The model under review builds one solid part; all positions refer to its coordinate system, in mm. Round coordinates to 2 decimals unless told otherwise and drop trailing zeros. Loops run counter-clockwise (first coordinate to the right, second up) from the corner with the lowest first, then second, coordinate; pieces in that order, holes last. Notation, with made-up numbers: (42.5, 50) -> (83.5, 50) arc R22 ccw to (83.5, 60) -> close; hole circle Ø9 at (64, -6). An arc over 180 degrees is marked (long way). Use a Markdown table: item, result. Add a question column.
1) Wall thickness on probe 1 along Z at (x, y) = (0, -12.25) (3 decimals); probe 2 along X at (y, z) = (-10.5, -21); probe 3 along Y at (x, z) = (1.25, -22.5): over which ranges is each line inside the solid? List them lowest first.
2) Consider section A-A on y = -14.5. Give the boundary of the cut face in (x, z) (3 decimals).
3) Mouldability with a two-part tool opening along X and no side actions: class faces 1 (the cylindrical face through (0.33, -8.62, -23.48)), 2 (the flat face through (0, 0, 0)), 3 (the cylindrical face through (-1.34, -8.62, 18.89)), 4 (the flat face through (7.5, -24, 0)) as released by +X, released by -X, zero draft, split by the parting line, or undercut.
from build123d import *

# Parameters (mm, degrees)
SKETCH1_W             = 15
SKETCH1_H             = 50
BOSS_EXTRUDE1_DEPTH   = 30.875
FILLET1_R             = 2
M6_TAPPED_HOLE1_D     = 5
M6_TAPPED_HOLE1_DEPTH = 17
M6_TAPPED_HOLE1_TIP   = 1.502151548


with BuildPart() as part:
    # Sketch1 → Boss-Extrude1 (new, symmetric)
    with BuildSketch(Plane.XY):
        with Locations((0, -25)):
            Rectangle(SKETCH1_W, SKETCH1_H)
    extrude(amount=BOSS_EXTRUDE1_DEPTH, both=True)

    # Fillet1
    fillet1_edges = [part.edges().sort_by_distance(p)[0] for p in [
        (7.5, -50, 0),
    ]]
    fillet(fillet1_edges, radius=FILLET1_R)

    # M6 Tapped Hole1
    with Locations(Plane(origin=(0, 0, 0), x_dir=(1, 0, 0), z_dir=(0, 1, 0))):
        with Locations((0, 21), (0, -21)):
            Hole(M6_TAPPED_HOLE1_D / 2, depth=M6_TAPPED_HOLE1_DEPTH)
            with Locations((0, 0, -(M6_TAPPED_HOLE1_DEPTH + M6_TAPPED_HOLE1_TIP / 2))):  # 118° drill point
                Cone(0, M6_TAPPED_HOLE1_D / 2, M6_TAPPED_HOLE1_TIP, mode=Mode.SUBTRACT)


solid = part.part
Result set:
| question | item | result |
|---|---|---|
| 1 | probe 1 | -30.875 to -23.5, -18.5 to 18.5, 23.5 to 30.875 |
| 1 | probe 2 | -7.5 to -2.5, 2.5 to 7.5 |
| 1 | probe 3 | -50 to -17.33 |
| 2 | outline | (-7.5, -30.875) -> (7.5, -30.875) -> (7.5, 30.875) -> (-7.5, 30.875) -> close; hole circle Ø5 at (0, -21); hole circle Ø5 at (0, 21) |
| 3 | face 1 | undercut |
| 3 | face 2 | zero draft |
| 3 | face 3 | undercut |
| 3 | face 4 | released by +X |
